Check sheet for the modelled part. Datum: model origin and axes. Units: mm. A direction names the side the tool comes from. Give positions to 0.01 mm unless a question says otherwise; leave off trailing zeros. Write each loop counter-clockwise with the first axis right and the second up, starting at its lowest first coordinate (ties: lowest second). Pieces come first, ordered by that corner, then holes. Notation, with made-up numbers: (10.5, 59) -> (52.5, 59) arc R26 ccw to (52.5, 73) -> close; hole circle Ø4 at (78, -4). An arc over 180 degrees is marked (long way). Return JSON: item names as keys, results as strings.
from build123d import *

# Parameters (mm, degrees)
F0_W          = 130.06
F0_H          = 109.46
F1_DEPTH      = 4.77
F2_R          = 8.735
F3_DEPTH      = 65.03
F3_DEPTH_BACK = 65.03


with BuildPart() as f1:
    # F0 (on Front) → F1 (new body)
    with BuildSketch(Plane.XZ):
        Rectangle(F0_W, F0_H)
    extrude(amount=F1_DEPTH)

    # F2 (on Right) → F3 (join, two sides)
    with BuildSketch(Plane.YZ) as f3_sk:
        with Locations((7.71413, 49.009632)):
            Circle(F2_R)
    extrude(amount=F3_DEPTH)
    extrude(f3_sk.sketch, amount=-F3_DEPTH_BACK)


solid = f1.part
(1) Thickness scan on L1, parallel to Y at x = -34.5, z = 11; L2, parallel to Z at x = -31, y = -2.5; L3, parallel to Y at x = -34, z = 43 (3 decimals). Record the ranges inside material, lowest first.
Reply:
{"L1": "-4.77 to 0", "L2": "-54.73 to 54.73", "L3": "-4.77 to 0, 1.375 to 14.053"}
(2) Set-up check for faces 4 (the flat face through (-1, -2, 54.73)), 5 (the flat face through (-65.03, -2, 14)): record each of +Z, -Z, +X, -X, +Y, -Y from which the full face is reachable in a straight line by a thin tool's end or side.
Reply:
{"face 4": "+Z, +X, -X, -Y", "face 5": "+Z, -Z, -X, +Y, -Y"}
(3) Cross-section at B-B on y = -3. Enter the section's corners in (x, z), then the cut area to 3 significant figures.
Reply:
{"outline": "(-65.03, -54.73) -> (65.03, -54.73) -> (65.03, 54.73) -> (-65.03, 54.73) -> close", "area": "14,200 mm^2"}
(4) Cross-section at A-A on x = 16. Enter the section's corners in (y, z) (3 decimals).
Reply:
{"outline": "(-4.77, -54.73) -> (0, -54.73) -> (0, 44.912) arc R8.735 ccw (long way) to (0, 53.107) -> (0, 54.73) -> (-4.77, 54.73) -> close"}
(5) Cross-section at C-C on z = -7.5. Enter the section's corners in (x, y).
Reply:
{"outline": "(-65.03, -4.77) -> (65.03, -4.77) -> (65.03, 0) -> (-65.03, 0) -> close"}
(6) Release check for a two-part mould opening along Y. For faces 1 (the cylindrical face through (0.91, 16.443, 48.685)), 2 (the flat face through (-1, -4.77, 1)), 3 (the flat face through (-1, -2, -54.73)) record: pulls with the +Y half, pulls with the -Y half, needs draft (parallel to the pull), parting line crosses it, or undercut.
Reply:
{"face 1": "undercut", "face 2": "pulls with the -Y half", "face 3": "needs draft"}
(7) Depth check by flat-ended pin: pin 1 Ø1.3 at (x, z) = (-21.5, 54) entering from +Y; pin 2 Ø10 at (x, y) = (-26.5, -1.5) entering from +Z; pin 3 Ø1.5 at (x, y) = (-5, 7.5) entering from -Z; pin 4 Ø8 at (y, z) = (5.5, -15) entering from +X. Enter the tip coordinate at first touch or a pass-through.
Reply:
{"pin 1": "y = 15.29", "pin 2": "z = 56.66", "pin 3": "z = 40.27", "pin 4": "through"}
